```python
from build123d import *

# Parameters (mm, degrees)
SKETCH_W        = 120
SKETCH_H        = 80
PAD_DEPTH       = 5
SKETCH001_R     = 1.5
POCKET_DEPTH    = 3
SKETCH002_R     = 2.85
POCKET001_DEPTH = 3
FILLET_R        = 1
PAD001_DEPTH    = 3


with BuildPart() as part:
    # Sketch → Pad (new body)
    with BuildSketch(Plane.XY):
        Rectangle(SKETCH_W, SKETCH_H)
    extrude(amount=PAD_DEPTH)

    # Sketch001 (on Face5 of Pad) → Pocket (cut)
    with BuildSketch(Plane(origin=(0, 0, 0), x_dir=(1, 0, 0), z_dir=(0, 0, -1))):
        with Locations((56, 36)):
            Circle(SKETCH001_R)
        with Locations((56, -36)):
            Circle(SKETCH001_R)
        with Locations((-56, 36)):
            Circle(SKETCH001_R)
        with Locations((-56, -36)):
            Circle(SKETCH001_R)
        Polygon((56.1, 29.6), (49.6, 36.1), (-49.6, 36.1), (-56.1, 29.6), (-56.1, -29.6), (-49.6, -36.1), (49.6, -36.1), (56.1, -29.6), align=None)
    extrude(amount=-POCKET_DEPTH, mode=Mode.SUBTRACT)

    # Sketch002 (on Face5 of Pocket) → Pocket001 (cut)
    with BuildSketch(Plane.XY.offset(5)):
        with Locations((56, 36)):
            Circle(SKETCH002_R)
        with Locations((56, -36)):
            Circle(SKETCH002_R)
        with Locations((-56, 36)):
            Circle(SKETCH002_R)
        with Locations((-56, -36)):
            Circle(SKETCH002_R)
    extrude(amount=-POCKET001_DEPTH, mode=Mode.SUBTRACT)

    # Fillet
    fillet_edges = [part.edges().sort_by_distance(p)[0] for p in [
        (60, -40, 2.5),
        (0, -40, 5),
        (-60, -40, 2.5),
        (-60, 0, 5),
        (0, 40, 5),
        (60, 0, 5),
        (60, 40, 2.5),
        (-60, 40, 2.5),
    ]]
    fillet(fillet_edges, radius=FILLET_R)

    # CopySketch003 → Pad001 (join)
    with BuildSketch(Plane(origin=(0, 0, 3), x_dir=(1, 0, 0), z_dir=(0, 0, -1))):
        Polygon((-48.9, 33.9), (48.9, 33.9), (53.9, 28.9), (53.9, -28.9), (48.9, -33.9), (-48.9, -33.9), (-53.9, -28.9), (-53.9, 28.9), align=None)
        Polygon((-48.2, 31.8), (48.2, 31.8), (51.8, 28.2), (51.8, -28.2), (48.2, -31.8), (-48.2, -31.8), (-51.8, -28.2), (-51.8, 28.2), align=None, mode=Mode.SUBTRACT)
    extrude(amount=PAD001_DEPTH)


solid = part.part
```
For this review, take the finished solid that the model builds, in its own axes (mm). A direction names the side the tool comes from. Give positions to 0.01 mm unless a question says otherwise; leave off trailing zeros. Write each loop counter-clockwise with the first axis right and the second up, starting at its lowest first coordinate (ties: lowest second). Pieces come first, ordered by that corner, then holes.
Item 1: Machinability: for faces 5 (the face through (-60, -1, 2)), 6 (the face through (56.1, 0, 1)), 7 (the face through (-54.685, -38.528, 3.521)), which of the approach directions +Z, -Z, +X, -X, +Y, -Y give a long, thin tool a straight path to every point of the face, cutting with its end or side? Answer none if there is none.
Item 2: The part is to be moulded in two halves that separate along Y. For faces 1 (the face through (51.4, -31.4, 1.5)), 2 (the face through (-1, -40, 2)), 3 (the face through (1, 33.9, 2)), 4 (the face through (-1, 1, 5)), say which applies: +Y half, -Y half, draft (parallel to the pull), parting line (faces both ways), or undercut.
Item 3: Take a section at B-B (x = -30). Give the boundary of the cut face in (y, z), and give its area (3 significant figures).
Item 4: Insertion check: P1, Ø4, axis at x = -56, y = -36, coming from the -Z side; P2, Ø2.5, axis at x = 56, y = 36, coming from the -Z side; P3, Ø5, axis at x = 12.5, y = 1, coming from the -Z side. Each pin has a flat end and moves straight along its axis. Give the tip position at first contact, or say it passes through.
Item 5: Wall thickness on probe 1 along Y at (x, z) = (-33, 2.95); probe 2 along X at (y, z) = (-22.5, 2.25); probe 3 along Y at (x, z) = (-56, 3.05): over which ranges is each line inside the solid? List them lowest first.
Item 6: Take a section at A-A (y = 9). Give the boundary of the cut face in (x, z), and give its area (3 significant figures).
Established:
1. face 5: +Z, -Z, -X, +Y, -Y
1. face 6: -Z
1. face 7: +Z
2. face 1: undercut
2. face 2: -Y half
2. face 3: undercut
2. face 4: draft
3. outline: (-40, 0) - (-36.1, 0) - (-36.1, 3) - (-33.9, 3) - (-33.9, 0) - (-31.8, 0) - (-31.8, 3) - (31.8, 3) - (31.8, 0) - (33.9, 0) - (33.9, 3) - (36.1, 3) - (36.1, 0) - (40, 0) - (40, 4) arc R1 ccw to (39, 5) - (-39, 5) arc R1 ccw to (-40, 4) - close
3. area: 196 mm2
4. P1: stops at z = 0
4. P2: passes through
4. P3: stops at z = 3
5. probe 1: y = -40 to -36.1, -33.9 to -31.8, 31.8 to 33.9, 36.1 to 40
5. probe 2: x = -60 to -56.1, -53.9 to -51.8, 51.8 to 53.9, 56.1 to 60
5. probe 3: y = -40 to -38.85, -33.15 to 33.15, 38.85 to 40
6. outline: (-60, 0) - (-56.1, 0) - (-56.1, 3) - (-53.9, 3) - (-53.9, 0) - (-51.8, 0) - (-51.8, 3) - (51.8, 3) - (51.8, 0) - (53.9, 0) - (53.9, 3) - (56.1, 3) - (56.1, 0) - (60, 0) - (60, 4) arc R1 ccw to (59, 5) - (-59, 5) arc R1 ccw to (-60, 4) - close
6. area: 276 mm2
